```python
from build123d import *

# Parameters (mm, degrees)
SKETCH_W    = 50
SKETCH_H    = 342
SKETCH003_R = 8.323834
SKETCH002_R = 15.87187


with BuildPart() as part:
    # Sketch → Revolution (revolve)
    with BuildSketch(Plane.XZ):
        with Locations((25, 171)):
            Rectangle(SKETCH_W, SKETCH_H)
    revolve(axis=Axis((0, 0, 0), (0, 0, 1)))

    # Sketch001 → Revolution001 (revolve)
    with BuildSketch(Plane.XZ):
        Polygon((50, 0), (38.572964, -28.773746), (38.572964, -33.573742), (29.993038, -33.573742), (29.993038, -38), (0, -38), (0, 0), align=None)
    revolve(axis=Axis((0, 0, 0), (0, 0, 1)))

    # Sketch003 (on DatumPlane) → SubtractiveLoft section 0
    with BuildSketch(Plane(origin=(0, 0, -8), x_dir=(1, 0, 0), z_dir=(0, 0, -1))):
        Circle(SKETCH003_R)
    # Sketch002 (on Face7 of Revolution001) → SubtractiveLoft section 1
    with BuildSketch(Plane(origin=(0, 0, -38), x_dir=(1, 0, 0), z_dir=(0, 0, -1))):
        Circle(SKETCH002_R)
    loft(mode=Mode.SUBTRACT)


solid = part.part
```
Could you check a few things on this model? Use its own coordinates, in mm. A direction names the side the tool comes from. Round coordinates to 2 decimals unless told otherwise and drop trailing zeros. Loops run counter-clockwise (first coordinate to the right, second up) from the corner with the lowest first, then second, coordinate; pieces in that order, holes last. Notation, with made-up numbers: (21.25, 60) -> (51.25, 60) arc R23 cw to (51.25, 81) -> close; hole circle Ø1 at (-4.75, -19.75). An arc over 180 degrees is marked (long way). One line per question, with ' | ' between items.
(1) Thinking about a two-plate mould opening in Y: for faces 3 (the face through (13, -13, -38)), 4 (the face through (37.32, 11.75, -27.38)), 5 (the face through (0, 0, -8)), which applies, released by +Y, released by -Y, zero draft, split by the parting line, or undercut?
Model answer:
face 3: zero draft | face 4: split by the parting line | face 5: undercut
(2) If we section it at B-B on z = 303: List the corners of the cut face in (x, y) for me.
Model answer:
outline: circle Ø100 at (0, 0)
(3) If we section it at A-A on x = 0: List the corners of the cut face in (y, z) for me.
Model answer:
outline: (-50, 0) -> (-38.57, -28.77) -> (-38.57, -33.57) -> (-29.99, -33.57) -> (-29.99, -38) -> (-15.87, -38) -> (-8.32, -8) -> (8.32, -8) -> (15.87, -38) -> (29.99, -38) -> (29.99, -33.57) -> (38.57, -33.57) -> (38.57, -28.77) -> (50, 0) -> (50, 342) -> (-50, 342) -> close
(4) If I drill on probe 1 along Z at (x, y) = (-5.5, -3); probe 2 along Y at (x, z) = (2, 196.5); probe 3 along Z at (x, y) = (32, 5.5), over which ranges is the centre line in solid material (lowest first)?
Model answer:
probe 1: z = -8 to 342 | probe 2: y = -49.96 to 49.96 | probe 3: z = -33.57 to 342
(5) For pin 1 Ø1.5 at (x, z) = (-0.5, 62.5) entering from +Y; pin 2 Ø1 at (x, z) = (-4, 82) entering from +Y; pin 3 Ø2 at (y, z) = (32.5, 89.5) entering from -X, each with a flat end and sliding along its axis, tell me the tip position at first contact or that it passes through.
Model answer:
pin 1: stops at y = 50 | pin 2: stops at y = 49.88 | pin 3: stops at x = -38.83
(6) For faces 1 (the face through (-5.021, 38.245, -31.207)), 2 (the face through (1, 1, 342)), which set-ups out of +Z, -Z, +X, -X, +Y, -Y let a thin tool reach every point of the face, with its end or its side?
Model answer:
face 1: -Z | face 2: +Z, +X, -X, +Y, -Y
